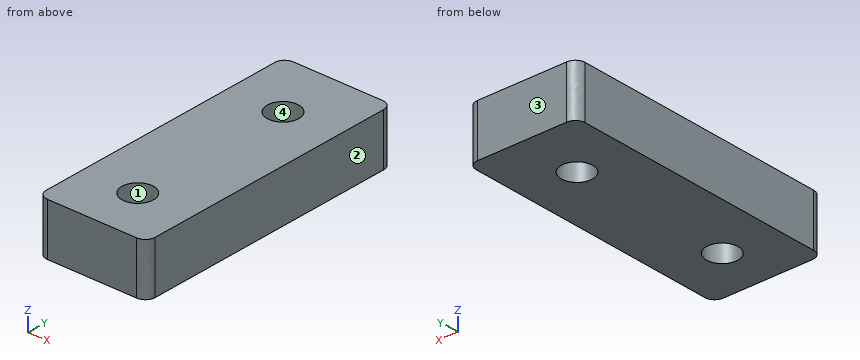
from build123d import *

# Parameters (mm, degrees)
MODEL_R             = 1.9243
MODEL_R_2           = 1.92515
BOSS_EXTRUDE1_DEPTH = 6.35


with BuildPart() as part:
    # Model → Boss-Extrude1 (new body)
    with BuildSketch(Plane.XY):
        with BuildLine():
            Line((-255.7004, 141.5182), (-244.7908, 141.5182))
            add(Edge.make_bspline(
                [(-244.7908, 141.5182), (-244.1268, 141.5182), (-243.5919, 140.9838), (-243.5919, 140.3197)],
                knots=[0.111111111, 0.111111111, 0.111111111, 0.111111111, 0.222222222, 0.222222222, 0.222222222, 0.222222222], degree=3))
            Line((-243.5919, 140.3197), (-243.5919, 108.5737))
            add(Edge.make_bspline(
                [(-243.5919, 108.5737), (-243.5919, 107.9096), (-244.1268, 107.3747), (-244.7908, 107.3747)],
                knots=[0.333333333, 0.333333333, 0.333333333, 0.333333333, 0.444444444, 0.444444444, 0.444444444, 0.444444444], degree=3))
            Line((-244.7908, 107.3747), (-255.7004, 107.3747))
            add(Edge.make_bspline(
                [(-255.7004, 107.3747), (-256.3648, 107.3747), (-256.8997, 107.9096), (-256.8997, 108.5737)],
                knots=[0.555555556, 0.555555556, 0.555555556, 0.555555556, 0.666666667, 0.666666667, 0.666666667, 0.666666667], degree=3))
            Line((-256.8997, 108.5737), (-256.8997, 140.3197))
            add(Edge.make_bspline(
                [(-256.8997, 140.3197), (-256.8997, 140.9838), (-256.3648, 141.5182), (-255.7004, 141.5182)],
                knots=[0.777777778, 0.777777778, 0.777777778, 0.777777778, 1, 1, 1, 1], degree=3))
        make_face()
        with Locations((-250.245, 133.8944)):
            Circle(MODEL_R, mode=Mode.SUBTRACT)
        with Locations((-250.245, 113.71655)):
            Circle(MODEL_R_2, mode=Mode.SUBTRACT)
    extrude(amount=BOSS_EXTRUDE1_DEPTH)


solid = part.part
Input: part model. Units: mm. Frame: model coordinates. Face numbers are marked on the shaded views. Give positions to 0.01 mm unless a question says otherwise; leave off trailing zeros. Loops run counter-clockwise (first coordinate to the right, second up) from the corner with the lowest first, then second, coordinate; pieces in that order, holes last. Notation, with made-up numbers: M -4,21 L 4,21 A31 cw 4,56 Z; hole C -12.5,5 d8. An arc over 180 degrees is marked long. Use one line per item in the form item = value.
1. First-contact query: pin 1 (2.5 mm diameter, centred on x = -250.24, y = 113.72, fed in from +Z). Flat tip, straight axial feed; report the tip coordinate or a pass-through.
Numbers:
pin_1 = through
2. Section query B-B, the plane z = 1.5. Count the separate pieces of the cut face and the enclosed holes in it, and give its area (3 significant figures).
Numbers:
separate_pieces = 1
enclosed_holes = 2
area = 430 mm²
3. Pull-direction query (X, two-part tool) for the marked faces 1, 2, 3 and 4; classes: released by +X, released by -X, zero draft, split by the parting line, or undercut.
Numbers:
face_1 = undercut
face_2 = released by +X
face_3 = zero draft
face_4 = undercut
4. Section query A-A, the plane x = -250.25. Return the cut outline in (y, z), and give its area (3 significant figures).
Numbers:
outline = M 107.37,0 L 111.79,0 L 111.79,6.35 L 107.37,6.35 Z; M 115.64,0 L 131.97,0 L 131.97,6.35 L 115.64,6.35 Z; M 135.82,0 L 141.52,0 L 141.52,6.35 L 135.82,6.35 Z
area = 168 mm²
5. Line query: L1, parallel to Y at x = -250.25, z = 1.75; L2, parallel to Y at x = -249, z = 1.75; L3, parallel to X at y = 133, z = 3.5. Output: solid intervals per line, ascending.
Numbers:
L1 = 107.37 to 111.79, 115.64 to 131.97, 135.82 to 141.52
L2 = 107.37 to 112.25, 115.18 to 132.43, 135.36 to 141.52
L3 = -256.9 to -251.95, -248.54 to -243.59
